from build123d import *

# Parameters (mm, degrees)
SKETCH1_W           = 500
SKETCH1_H           = 150
BOSS_EXTRUDE1_DEPTH = 50
SKETCH2_W           = 15.384615385
SKETCH2_H           = 15.384615384
SKETCH2_W_2         = 15.384615384
SKETCH2_H_2         = 80
CUT_EXTRUDE1_DEPTH  = 20
SKETCH3_R           = 10
CUT_EXTRUDE2_DEPTH  = 266.753645441
CHAMFER1_SIZE       = 4


with BuildPart() as part:
    # Sketch1 → Boss-Extrude1 (new body)
    with BuildSketch(Plane(origin=(0, 0, 0), x_dir=(1, 0, 0), z_dir=(0, 1, 0))):
        Rectangle(SKETCH1_W, SKETCH1_H)
    extrude(amount=BOSS_EXTRUDE1_DEPTH)

    # Sketch2 → Cut-Extrude1 (cut)
    # profile 1 of 8: a face of its own
    with BuildSketch(Plane(origin=(0, 50, 0), x_dir=(1, 0, 0), z_dir=(0, 1, 0))):
        with BuildLine():
            Line((-220.114547961, -33.307849889), (-220.114547961, 46.692150111))
            Line((-220.114547961, 46.692150111), (-194.521599243, 46.692150111))
            add(Edge.make_bspline(
                [(-194.521599243, 46.692150111), (-193.362373318, 46.690884181), (-191.145215926, 46.68846294), (-187.982575017, 46.621190731), (-185.135090695, 46.525959504), (-182.606989081, 46.407353042), (-180.389374452, 46.23036942), (-178.492194776, 46.025425049), (-176.903503637, 45.804959291), (-175.967970488, 45.576806717), (-175.547240269, 45.474201393)],
                knots=[0, 0, 0, 0, 1.460485487, 2.793352117, 3.985295279, 5.050041172, 5.981765236, 6.787433016, 7.454681457, 8, 8, 8, 8], degree=3))
            add(Edge.make_bspline(
                [(-175.547240269, 45.474201393), (-174.987771388, 45.314675255), (-173.877356736, 44.998053247), (-172.286478808, 44.323065419), (-170.753124402, 43.540790537), (-169.296558471, 42.608460279), (-167.911829693, 41.542626797), (-166.594822019, 40.351982104), (-165.338512035, 39.03115138), (-164.160279176, 37.582743847), (-163.081156481, 36.014063129), (-162.148523341, 34.322789965), (-161.367171772, 32.516275498), (-160.701473221, 30.608095458), (-160.210317655, 28.577791061), (-159.866598053, 26.439469094), (-159.627326323, 24.1921943), (-159.610385144, 22.654342715), (-159.601727448, 21.868432162)],
                knots=[0, 0, 0, 0, 0.907145743, 1.80047177, 2.69161667, 3.591261238, 4.495029544, 5.415863088, 6.359363025, 7.337192411, 8.326890979, 9.326929023, 10.346104993, 11.395420813, 12.477187422, 13.601053412, 14.774031606, 16, 16, 16, 16], degree=3))
            add(Edge.make_bspline(
                [(-159.601727448, 21.868432162), (-159.626419152, 20.674937637), (-159.673952037, 18.377395143), (-160.205760683, 15.083589507), (-161.016899695, 12.074910394), (-162.202437968, 9.380337629), (-163.647855404, 6.989297258), (-165.240012468, 4.833785656), (-167.058021858, 2.978772131), (-169.022220631, 1.394320163), (-171.098019744, 0.097670408), (-173.177576478, -1.007705098), (-175.288951411, -1.857553106), (-176.728482139, -2.227838717), (-177.43826591, -2.410413992)],
                knots=[0, 0, 0, 0, 1.312386234, 2.526415563, 3.661883817, 4.733421185, 5.753802465, 6.732107337, 7.675884281, 8.604170108, 9.50284679, 10.365392406, 11.194030444, 12, 12, 12, 12], degree=3))
            add(Edge.make_bspline(
                [(-177.43826591, -2.410413992), (-177.944874755, -2.5067829), (-179.012745754, -2.70991706), (-180.706325278, -2.912404846), (-182.557499482, -3.136536749), (-184.573882373, -3.282728169), (-186.753034651, -3.419630304), (-189.094110145, -3.484266322), (-191.593763206, -3.562139599), (-193.314257132, -3.563538884), (-194.201086423, -3.564260146)],
                knots=[0, 0, 0, 0, 0.735353946, 1.55003838, 2.431865514, 3.394945452, 4.432993119, 5.54609699, 6.735134699, 8, 8, 8, 8], degree=3))
            Line((-194.201086423, -3.564260146), (-204.729932576, -3.564260146))
            Line((-204.729932576, -3.564260146), (-204.729932576, -33.307849889))
            Line((-204.729932576, -33.307849889), (-220.114547961, -33.307849889))
        make_face()
        with BuildLine():
            Line((-204.729932576, 33.358816777), (-204.729932576, 9.769073188))
            Line((-204.729932576, 9.769073188), (-195.499163346, 9.769073188))
            add(Edge.make_bspline(
                [(-195.499163346, 9.769073188), (-194.703153264, 9.770103954), (-193.180285827, 9.772075938), (-190.995308866, 9.842858626), (-189.017465651, 9.929262023), (-187.242623546, 10.072277323), (-185.681495968, 10.26076807), (-184.32362843, 10.486226744), (-183.167438366, 10.728167456), (-181.917176214, 11.129101986), (-180.580396005, 11.777777497), (-179.152871842, 12.710087135), (-177.89879355, 13.824773264), (-176.855234189, 15.133933521), (-176.021661303, 16.588486417), (-175.42482251, 18.173525213), (-175.039444262, 19.862780272), (-175.004243472, 21.03297104), (-174.986342833, 21.628047547)],
                knots=[0, 0, 0, 0, 1.411705958, 2.700771114, 3.876961699, 4.922619712, 5.858038221, 6.66485904, 7.363650596, 7.950905807, 8.989198271, 9.987739806, 10.967313358, 11.951275539, 12.944273208, 13.927870418, 14.946261014, 16, 16, 16, 16], degree=3))
            add(Edge.make_bspline(
                [(-174.986342833, 21.628047547), (-175.011536019, 22.35284144), (-175.060382286, 23.758121234), (-175.599020255, 25.759474192), (-176.43007709, 27.575726264), (-177.618252422, 29.15036565), (-179.053540257, 30.474507882), (-180.666743883, 31.576241297), (-182.492313993, 32.347242727), (-183.784328311, 32.645977321), (-184.441471038, 32.797919342)],
                knots=[0, 0, 0, 0, 1.085904563, 2.105425768, 3.088705091, 4.068969419, 5.045188284, 6.010769642, 6.988240112, 8, 8, 8, 8], degree=3))
            add(Edge.make_bspline(
                [(-184.441471038, 32.797919342), (-184.724254567, 32.843148261), (-185.351946325, 32.94354244), (-186.39529777, 33.048316251), (-187.629582692, 33.143607927), (-189.056288904, 33.22184524), (-190.669761298, 33.283008702), (-192.475321832, 33.33660298), (-194.468215217, 33.340908569), (-195.862424259, 33.352681985), (-196.588906935, 33.358816777)],
                knots=[0, 0, 0, 0, 0.564603001, 1.253243608, 2.066786758, 3.005752288, 4.070476343, 5.250658742, 6.567396469, 8, 8, 8, 8], degree=3))
            Line((-196.588906935, 33.358816777), (-204.729932576, 33.358816777))
        make_face(mode=Mode.SUBTRACT)
    # profile 2 of 8: a face of its own
    with BuildSketch(Plane(origin=(0, 50, 0), x_dir=(1, 0, 0), z_dir=(0, 1, 0))):
        with Locations((-138.576086422, -25.615542197)):
            Rectangle(SKETCH2_W, SKETCH2_H)
    # profile 3 of 8: a face of its own
    with BuildSketch(Plane(origin=(0, 50, 0), x_dir=(1, 0, 0), z_dir=(0, 1, 0))):
        Polygon((-97.037624884, -33.307849889), (-97.037624884, 33.358816777), (-120.627368474, 33.358816777), (-120.627368474, 46.692150111), (-58.06326591, 46.692150111), (-58.06326591, 33.358816777), (-81.653009499, 33.358816777), (-81.653009499, -33.307849889), align=None)
    # profile 4 of 8: a face of its own
    with BuildSketch(Plane(origin=(0, 50, 0), x_dir=(1, 0, 0), z_dir=(0, 1, 0))):
        with Locations((-40.114547961, -25.615542197)):
            Rectangle(SKETCH2_W_2, SKETCH2_H)
    # profile 5 of 8: a face of its own
    with BuildSketch(Plane(origin=(0, 50, 0), x_dir=(1, 0, 0), z_dir=(0, 1, 0))):
        Polygon((1.423913577, -33.307849889), (1.423913577, 33.358816777), (-22.165830012, 33.358816777), (-22.165830012, 46.692150111), (40.398272552, 46.692150111), (40.398272552, 33.358816777), (16.808528962, 33.358816777), (16.808528962, -33.307849889), align=None)
    # profile 6 of 8: a face of its own
    with BuildSketch(Plane(origin=(0, 50, 0), x_dir=(1, 0, 0), z_dir=(0, 1, 0))):
        with Locations((57.321349475, 6.692150111)):
            Rectangle(SKETCH2_W_2, SKETCH2_H_2)
    # profile 7 of 8: a face of its own
    with BuildSketch(Plane(origin=(0, 50, 0), x_dir=(1, 0, 0), z_dir=(0, 1, 0))):
        Polygon((81.423913577, -33.307849889), (81.423913577, 46.692150111), (140.911093065, 46.692150111), (140.911093065, 33.358816777), (96.808528962, 33.358816777), (96.808528962, 15.922919342), (137.834169988, 15.922919342), (137.834169988, 2.589586008), (96.808528962, 2.589586008), (96.808528962, -19.974516556), (141.93673409, -19.974516556), (141.93673409, -33.307849889), align=None)
    # profile 8 of 8: a face of its own
    with BuildSketch(Plane(origin=(0, 50, 0), x_dir=(1, 0, 0), z_dir=(0, 1, 0))):
        Polygon((155.270067424, -33.307849889), (155.270067424, 46.692150111), (171.343785372, 46.692150111), (203.475195629, -5.904003735), (203.475195629, 46.692150111), (218.859811013, 46.692150111), (218.859811013, -33.307849889), (202.289298193, -33.307849889), (170.654682808, 18.454970624), (170.654682808, -33.307849889), align=None)
    extrude(amount=-CUT_EXTRUDE1_DEPTH, mode=Mode.SUBTRACT)

    # Sketch3 → Cut-Extrude2 (cut, through all)
    with BuildSketch(Plane(origin=(0, 50, 0), x_dir=(1, 0, 0), z_dir=(0, 1, 0))):
        with Locations(Location((-230, 60, 0), (0, 0, 270))):
            Circle(SKETCH3_R)
        with Locations(Location((-230, -60, 0), (0, 0, 270))):
            Circle(SKETCH3_R)
        with Locations(Location((230, -60, 0), (0, 0, 270))):
            Circle(SKETCH3_R)
        with Locations(Location((230, 60, 0), (0, 0, 270))):
            Circle(SKETCH3_R)
    extrude(amount=-CUT_EXTRUDE2_DEPTH, mode=Mode.SUBTRACT)

    # Chamfer1
    chamfer1_edges = [part.edges().sort_by_distance(p)[0] for p in [
        (-250, 50, 0),
        (0, 50, 75),
        (250, 50, 0),
        (0, 50, -75),
    ]]
    chamfer(chamfer1_edges, length=CHAMFER1_SIZE)


solid = part.part
CAD build for the part. Positions are in the model's coordinates, mm. A direction names the side the tool comes from. Coordinates: 2 decimals unless noted, no trailing zeros. Write each loop counter-clockwise with the first axis right and the second up, starting at its lowest first coordinate (ties: lowest second). Pieces come first, ordered by that corner, then holes. Notation, with made-up numbers: M -35.5,5 L -13.5,5 A33 ccw -13.5,38 Z; hole C 80.5,-11.75 d4. An arc over 180 degrees is marked long. Answer as a JSON object with one key per item and string values. Group by question number.
1) Saw through at D-D (x = 230). Write the cut outline in (y, z).
2) Mould opens along Z. For faces 3 (the face through (-204.73, 40, -22)), 4 (the face through (-250, 23, 1)), 5 (the face through (-97.038, 40, 0)) say: +Z half, -Z half, draft (parallel to the pull), parting line (faces both ways), or undercut.
3) Saw through at C-C (y = 7). Write the cut outline in (x, z).
4) Saw through at B-B (x = 162). Write the cut outline in (y, z), plus the area to 3 significant figures.
5) Tool access for faces 1 (the face through (170.655, 40, 7)), 2 (the face through (236.76, 25.35, -67.37)): list every direction of +Z, -Z, +X, -X, +Y, -Y with a clear straight run to the whole face (end or side of a thin tool).
6) Pin check, flat tip, straight feed: pin 1 Ø1.5 at (x, z) = (188.5, -16.5) entering from +Y. Stop position of the tip, or through.
7) Wall check: line 1 (X direction, y = 26, z = -60); line 2 (Z direction, x = 162, y = 44); line 3 (Y direction, x = 52, z = 31.5). Give the ranges that are in metal, low to high. Write a range as from..to.
8) Saw through at A-A (z = 60). Write the cut outline in (x, y), plus the area to 3 significant figures.
Values follow:
{
 "1": {"outline": "M 0,-75 L 46,-75 L 50,-71 L 50,-70 L 0,-70 Z; M 0,-50 L 50,-50 L 50,50 L 0,50 Z; M 0,70 L 50,70 L 50,71 L 46,75 L 0,75 Z"},
 "2": {"face 3": "undercut", "face 4": "draft", "face 5": "undercut"},
 "3": {"outline": "M -250,-75 L 250,-75 L 250,75 L -250,75 Z; hole C -230,-60 d20; hole C -230,60 d20; hole C 230,-60 d20; hole C 230,60 d20"},
 "4": {"outline": "M 0,-75 L 46,-75 L 50,-71 L 50,-46.69 L 30,-46.69 L 30,33.31 L 50,33.31 L 50,71 L 46,75 L 0,75 Z", "area": "5,880 mm2"},
 "5": {"face 1": "+Y", "face 2": "+Y, -Y"},
 "6": {"pin 1": "stops at y = 30"},
 "7": {"line 1": "x = -250..-240, -220..220, 240..250", "line 2": "z = -75..-46.69, 33.31..75", "line 3": "y = 0..30"},
 "8": {"outline": "M -250,0 L -240,0 L -240,50 L -246,50 L -250,46 Z; M -220,0 L 220,0 L 220,50 L -220,50 Z; M 240,0 L 250,0 L 250,46 L 246,50 L 240,50 Z", "area": "23,000 mm2"}
}
